from build123d import *

# Parameters (mm, degrees)
BOSS_EXTRUDE1_DEPTH     = 12.7
CUT_EXTRUDE1_DEPTH      = 55.824592329
CUT_EXTRUDE1_DEPTH_BACK = 55.824592329
SKETCH3_R               = 2.54


with BuildPart() as part:
    # Sketch1 → Boss-Extrude1 (new body)
    with BuildSketch(Plane(origin=(0, 0, 0), x_dir=(1, 0, 0), z_dir=(0, 1, 0))):
        Polygon((0, 0), (24.384, 0), (24.384, 11.43), (21.59, 11.43), (21.59, 8.89), (8.89, 8.89), (8.89, 21.59), (0, 21.59), align=None)
    boss_extrude1 = extrude(amount=BOSS_EXTRUDE1_DEPTH)

    # Mirror1: Boss-Extrude1 across plane
    add(boss_extrude1.mirror(Plane(origin=(24.384, 12.7, -11.43), x_dir=(0, 0, 1), z_dir=(-1, 0, 0))))

    # Sketch3 → Cut-Extrude1 (cut, two sides: drawn at the far end of the back side and taken through both)
    with BuildSketch(Plane.ZY.offset(-CUT_EXTRUDE1_DEPTH_BACK)):
        with Locations((-15.24, 6.35)):
            Circle(SKETCH3_R)
    extrude(amount=CUT_EXTRUDE1_DEPTH + CUT_EXTRUDE1_DEPTH_BACK, mode=Mode.SUBTRACT)


solid = part.part
Build history of the part. All positions in model axes, mm. A direction names the side the tool comes from. Coordinates: 2 decimals unless noted, no trailing zeros. Write each loop counter-clockwise with the first axis right and the second up, starting at its lowest first coordinate (ties: lowest second). Pieces come first, ordered by that corner, then holes.
(1) 3-axis set-ups, long thin cutter, end or side, ignore diameter. For faces 4 (the flat face through (24, 6, -11.43)), 5 (the flat face through (48.768, 6, -11)): which of +Z, -Z, +X, -X, +Y, -Y reach the whole face in a straight line?
(2) Cut at C-C on z = -9.75. List the corners of the cut face in (x, y), and give its area (3 significant figures).
(3) Cut at A-A on z = -15.24. List the corners of the cut face in (x, y).
(4) Cut at B-B on y = 6.35. List the corners of the cut face in (x, z), and give its area (3 significant figures).
(5) Cut at D-D on y = 12. List the corners of the cut face in (x, z).
(6) Drill centre lines: line 1 (X direction, y = 12.25, z = -10); line 2 (X direction, y = 2, z = -13); line 3 (Z direction, x = 2.75, y = 6.35). Where is each one in solid material? Low to high.
(7) Mould opens along X. For faces 1 (the flat face through (27.178, 6, -10)), 2 (the flat face through (0, 6, -11)), 3 (the flat face through (25, 12.7, -9)) say: pulls with the +X half, pulls with the -X half, needs draft (parallel to the pull), parting line crosses it, or undercut.
(8) Pin check, flat tips, straight feed: pin 1 Ø1.7 at (x, y) = (25, 6.5) entering from -Z; pin 2 Ø3 at (y, z) = (6.35, -15.24) entering from -X; pin 3 Ø4 at (x, y) = (13, 4) entering from -Z. Stop position of each tip, or through.
Working result:
1. face 4: -Z, +Y, -Y
1. face 5: +Z, -Z, +X, +Y, -Y
2. outline: (0, 0) - (8.89, 0) - (8.89, 12.7) - (0, 12.7) - close; (21.59, 0) - (27.18, 0) - (27.18, 12.7) - (21.59, 12.7) - close; (39.88, 0) - (48.77, 0) - (48.77, 12.7) - (39.88, 12.7) - close
2. area: 297 mm2
3. outline: (0, 0) - (8.89, 0) - (8.89, 3.81) - (0, 3.81) - close; (0, 8.89) - (8.89, 8.89) - (8.89, 12.7) - (0, 12.7) - close; (39.88, 0) - (48.77, 0) - (48.77, 3.81) - (39.88, 3.81) - close; (39.88, 8.89) - (48.77, 8.89) - (48.77, 12.7) - (39.88, 12.7) - close
4. outline: (0, -21.59) - (8.89, -21.59) - (8.89, -17.78) - (0, -17.78) - close; (0, -12.7) - (8.89, -12.7) - (8.89, -8.89) - (21.59, -8.89) - (21.59, -11.43) - (27.18, -11.43) - (27.18, -8.89) - (39.88, -8.89) - (39.88, -12.7) - (48.77, -12.7) - (48.77, 0) - (0, 0) - close; (39.88, -21.59) - (48.77, -21.59) - (48.77, -17.78) - (39.88, -17.78) - close
4. area: 583 mm2
5. outline: (0, -21.59) - (8.89, -21.59) - (8.89, -8.89) - (21.59, -8.89) - (21.59, -11.43) - (27.18, -11.43) - (27.18, -8.89) - (39.88, -8.89) - (39.88, -21.59) - (48.77, -21.59) - (48.77, 0) - (0, 0) - close
6. line 1: x = 0 to 8.89, 21.59 to 27.18, 39.88 to 48.77
6. line 2: x = 0 to 8.89, 39.88 to 48.77
6. line 3: z = -21.59 to -17.78, -12.7 to 0
7. face 1: undercut
7. face 2: pulls with the -X half
7. face 3: needs draft
8. pin 1: stops at z = -11.43
8. pin 2: passes through
8. pin 3: stops at z = -8.89
